Design review of the part built by this model. Coordinates are the model's own, in mm. A direction names the side the tool comes from. Give positions to 0.01 mm unless a question says otherwise; leave off trailing zeros. Loops run counter-clockwise (first coordinate to the right, second up) from the corner with the lowest first, then second, coordinate; pieces in that order, holes last. Notation, with made-up numbers: (84.25, 18.25) - (129.25, 18.25) arc R19 ccw to (129.25, 29.25) - close; hole circle Ø6 at (-24, 21). An arc over 180 degrees is marked (long way). Write each question's results on one line, items separated by ' | '.
from build123d import *

# Parameters (mm, degrees)
SKETCH1_W           = 15
SKETCH1_H           = 70
BOSS_EXTRUDE1_DEPTH = 8
SKETCH2_W           = 1
SKETCH2_H           = 50
CUT_EXTRUDE1_DEPTH  = 8
SKETCH3_R           = 2.5
CUT_EXTRUDE2_DEPTH  = 8
SKETCH4_R           = 2.75
CUT_EXTRUDE3_DEPTH  = 8
SKETCH5_R           = 5
CUT_EXTRUDE4_DEPTH  = 4.2


with BuildPart() as part:
    # Sketch1 → Boss-Extrude1 (new body)
    with BuildSketch(Plane(origin=(0, 0, 0), x_dir=(1, 0, 0), z_dir=(0, 1, 0))):
        Rectangle(SKETCH1_W, SKETCH1_H)
    extrude(amount=BOSS_EXTRUDE1_DEPTH)

    # Sketch2 → Cut-Extrude1 (cut)
    with BuildSketch(Plane(origin=(0, 8, 0), x_dir=(1, 0, 0), z_dir=(0, 1, 0))):
        with Locations((7, 0)):
            Rectangle(SKETCH2_W, SKETCH2_H)
    extrude(amount=-CUT_EXTRUDE1_DEPTH, mode=Mode.SUBTRACT)

    # Sketch3 → Cut-Extrude2 (cut)
    with BuildSketch(Plane(origin=(0, 8, 0), x_dir=(1, 0, 0), z_dir=(0, 1, 0))):
        with Locations((-0.5, -29)):
            Circle(SKETCH3_R)
        with Locations((-0.5, 29)):
            Circle(SKETCH3_R)
    extrude(amount=-CUT_EXTRUDE2_DEPTH, mode=Mode.SUBTRACT)

    # Sketch4 → Cut-Extrude3 (cut)
    with BuildSketch(Plane(origin=(0, 8, 0), x_dir=(1, 0, 0), z_dir=(0, 1, 0))):
        with Locations((-0.5, -17.5)):
            Circle(SKETCH4_R)
        with Locations((-0.5, 17.5)):
            Circle(SKETCH4_R)
    extrude(amount=-CUT_EXTRUDE3_DEPTH, mode=Mode.SUBTRACT)

    # Sketch5 → Cut-Extrude4 (cut)
    with BuildSketch(Plane(origin=(0, 8, 0), x_dir=(1, 0, 0), z_dir=(0, 1, 0))):
        with Locations((-0.5, 17.5)):
            Circle(SKETCH5_R)
        with Locations((-0.5, -17.5)):
            Circle(SKETCH5_R)
    extrude(amount=-CUT_EXTRUDE4_DEPTH, mode=Mode.SUBTRACT)


solid = part.part
(1) Take a section at A-A on z = -17.5. Give the boundary of the cut face in (x, y).
Answers below:
outline: (-7.5, 0) - (-3.25, 0) - (-3.25, 3.8) - (-5.5, 3.8) - (-5.5, 8) - (-7.5, 8) - close; (2.25, 0) - (6.5, 0) - (6.5, 8) - (4.5, 8) - (4.5, 3.8) - (2.25, 3.8) - close
(2) Draft analysis for pull direction Z (two halves, no side actions). For faces 1 (the flat face through (0, 4, -35)), 2 (the flat face through (2, 3.8, 20)), 3 (the cylindrical face through (-0.83, 4.06, 26.52)), 4 (the flat face through (0, 4, 35)), state which applies: pulls with the +Z half, pulls with the -Z half, needs draft (parallel to the pull), parting line crosses it, or undercut.
Answers below:
face 1: pulls with the -Z half | face 2: undercut | face 3: undercut | face 4: pulls with the +Z half
(3) Take a section at C-C on z = 29. Give the boundary of the cut face in (x, y).
Answers below:
outline: (-7.5, 0) - (-3, 0) - (-3, 8) - (-7.5, 8) - close; (2, 0) - (7.5, 0) - (7.5, 8) - (2, 8) - close
(4) Wall thickness on line 1 along Z through (x, y) = (-0.5, 3.5); line 2 along Z through (x, y) = (-0.5, 6.65); line 3 along Z through (x, y) = (3.25, 5.5): over which ranges is each line inside the solid? List them lowest first. Write a range as from..to.
Answers below:
line 1: -35..-31.5, -26.5..-20.25, -14.75..14.75, 20.25..26.5, 31.5..35 | line 2: -35..-31.5, -26.5..-22.5, -12.5..12.5, 22.5..26.5, 31.5..35 | line 3: -35..-20.81, -14.19..14.19, 20.81..35
(5) Tool access review of faces 5 (the cylindrical face through (-0.858, 1.927, -20.227)), 6 (the flat face through (6.5, 4, 0)), 7 (the cylindrical face through (-1.58, 5.93, -12.62)): name each direction out of +Z, -Z, +X, -X, +Y, -Y from which nothing blocks a thin tool from reaching the whole face with its end or side.
Answers below:
face 5: +Y, -Y | face 6: +X, +Y, -Y | face 7: +Y
(6) Insertion check: P1, Ø3, axis at x = -2.5, z = 17.5, coming from the +Y side; P2, Ø4.5, axis at x = -0.5, z = -17.5, coming from the -Y side. Each pin has a flat end and moves straight along its axis. Give the tip position at first contact, or say it passes through.
Answers below:
P1: y = 3.8 | P2: through
(7) Take a section at D-D on z = 15.5. Give the boundary of the cut face in (x, y), plus the area to 3 significant figures.
Answers below:
outline: (-7.5, 0) - (-2.39, 0) - (-2.39, 3.8) - (-5.08, 3.8) - (-5.08, 8) - (-7.5, 8) - close; (1.39, 0) - (6.5, 0) - (6.5, 8) - (4.08, 8) - (4.08, 3.8) - (1.39, 3.8) - close | area: 59.2 mm2
(8) Take a section at B-B on y = 6.25. Give the boundary of the cut face in (x, z).
Answers below:
outline: (-7.5, -35) - (7.5, -35) - (7.5, -25) - (6.5, -25) - (6.5, 25) - (7.5, 25) - (7.5, 35) - (-7.5, 35) - close; hole circle Ø10 at (-0.5, -17.5); hole circle Ø10 at (-0.5, 17.5); hole circle Ø5 at (-0.5, -29); hole circle Ø5 at (-0.5, 29)
